from build123d import *

# Parameters (mm, degrees)
BOSS_EXTRUDE1_DEPTH     = 14
SKETCH2_R               = 4
CUT_EXTRUDE1_DEPTH      = 42.386471219
SKETCH3_R               = 6
CUT_EXTRUDE2_DEPTH      = 0.5
CUT_EXTRUDE3_START      = -0.5
SKETCH4_R               = 6
CUT_EXTRUDE3_DEPTH      = 0.5
SKETCH5_R               = 2.5
CUT_EXTRUDE4_DEPTH      = 37.813584449
CUT_EXTRUDE5_REACH      = 43.386
CUT_EXTRUDE5_END_RADIUS = 4
SKETCH7_W               = 0.5
SKETCH7_H               = 14
FILLET1_R               = 2
FILLET2_R               = 0.5
FILLET3_R               = 0.25


with BuildPart() as part:
    # Sketch1 → Boss-Extrude1 (new body)
    with BuildSketch(Plane.XY):
        Polygon((21, 0), (-21, 0), (-21, 6), (-9, 6), (-9, 32.8), (9, 32.8), (9, 6), (21, 6), align=None)
    extrude(amount=BOSS_EXTRUDE1_DEPTH)

    # Sketch2 → Cut-Extrude1 (cut, through all)
    with BuildSketch(Plane.XY.offset(14)):
        with Locations((0, 20)):
            Circle(SKETCH2_R)
    extrude(amount=-CUT_EXTRUDE1_DEPTH, mode=Mode.SUBTRACT)

    # Sketch3 → Cut-Extrude2 (cut)
    with BuildSketch(Plane.XY.offset(14)):
        with Locations((0, 20)):
            Circle(SKETCH3_R)
    extrude(amount=-CUT_EXTRUDE2_DEPTH, mode=Mode.SUBTRACT)

    # Sketch4 → Cut-Extrude3 (cut)
    with BuildSketch(Plane(origin=(0, 0, 0), x_dir=(-1, 0, 0), z_dir=(0, 0, -1)).offset(CUT_EXTRUDE3_START)):
        with Locations(Location((0, 20, 0), (0, 0, 180))):
            Circle(SKETCH4_R)
    extrude(amount=CUT_EXTRUDE3_DEPTH, mode=Mode.SUBTRACT)

    # Sketch5 → Cut-Extrude4 (cut, through all)
    with BuildSketch(Plane(origin=(0, 6, 0), x_dir=(1, 0, 0), z_dir=(0, 1, 0))):
        with Locations(Location((-16, -7, 0), (0, 0, 270))):
            Circle(SKETCH5_R)
        with Locations(Location((16, -7, 0), (0, 0, 90))):
            Circle(SKETCH5_R)
    extrude(amount=-CUT_EXTRUDE4_DEPTH, mode=Mode.SUBTRACT)

    # Cut-Extrude5: up to this cylinder (the profile starts outside it)
    cut_extrude5_end = Plane(origin=(0, 20, 7), z_dir=(0, 0, 1)) * Cylinder(CUT_EXTRUDE5_END_RADIUS, 95.772, mode=Mode.PRIVATE)
    # Sketch7 → Cut-Extrude5 (cut, up to the surface)
    with BuildSketch(Plane(origin=(0, 32.8, 0), x_dir=(1, 0, 0), z_dir=(0, 1, 0)), mode=Mode.PRIVATE) as cut_extrude5_sk1:
        with Locations((0, -7)):
            Rectangle(SKETCH7_W, SKETCH7_H)
    cut_extrude5_tool1 = extrude(cut_extrude5_sk1.sketch, amount=-CUT_EXTRUDE5_REACH, mode=Mode.PRIVATE) - cut_extrude5_end
    add(cut_extrude5_tool1.solids().sort_by_distance((0, 32.8, 7))[0], mode=Mode.SUBTRACT)

    # Fillet1
    fillet1_edges = [part.edges().sort_by_distance(p)[0] for p in [
        (-9, 6, 7),
        (9, 6, 7),
    ]]
    fillet(fillet1_edges, radius=FILLET1_R)

    # Fillet2
    fillet2_edges = [part.edges().sort_by_distance(p)[0] for p in [
        (-9, 32.8, 7),
        (9, 32.8, 7),
        (21, 6, 7),
        (-21, 6, 7),
        (-0.25, 32.8, 7),
        (0.25, 32.8, 7),
    ]]
    fillet(fillet2_edges, radius=FILLET2_R)

    # Fillet3
    fillet3_edges = [part.edges().sort_by_distance(p)[0] for p in [
        (-16, 6, 4.5),
        (16, 6, 9.5),
    ]]
    fillet(fillet3_edges, radius=FILLET3_R)


solid = part.part
Geometry: final body of the model. Coordinates: model frame, mm. A direction names the side the tool comes from. Round coordinates to 2 decimals unless told otherwise and drop trailing zeros. Loops run counter-clockwise (first coordinate to the right, second up) from the corner with the lowest first, then second, coordinate; pieces in that order, holes last.
Q1. Pin query (flat end, axial travel): P1, Ø13, axis at x = 0, y = 20, coming from the -Z side; P2, Ø3, axis at x = -17, z = 10, coming from the +Y side; P3, Ø6.5, axis at y = 29.5, z = 6.5, coming from the +X side; P4, Ø11, axis at x = 0, y = 20, coming from the +Z side. Return the tip coordinate at first contact, or that it passes through.
Q2. Section D-D on z = 1.25. Return loops of the section in (x, y).
Q3. Material intervals for L1, parallel to X at y = 1.9, z = 7; L2, parallel to X at y = 20, z = 0.4; L3, parallel to X at y = 20, z = 5.25, sorted ascending.
Q4. Pull-direction query (Z, two-part tool) for faces 4 (the cylindrical face through (-16.96, 2.92, 9.31)), 5 (the flat face through (5, 32.8, 7)), 6 (the flat face through (0, 9, 14)); classes: released by +Z, released by -Z, zero draft, split by the parting line, or undercut.
Q5. Access query for faces 1 (the flat face through (-16, 6, 4)), 2 (the flat face through (9, 20, 7)), 3 (the flat face through (-1.42, 16.08, 13.5)). Directions: +Z, -Z, +X, -X, +Y, -Y. A direction counts if a zero-diameter tool reaches every point of the face in a straight line with its end or side. Return the directions, or none.
Q6. Section B-B on z = 7. State how many separate pieces and enclosed holes the cut face has, plus the area to 3 significant figures.
Q7. Section A-A on y = 29. Return loops of the section in (x, z), plus the area to 3 significant figures.
Q8. Section C-C on x = -16. Return loops of the section in (y, z).
Evaluation:
1. P1: stops at z = 0
1. P2: stops at y = 6
1. P3: stops at x = 9
1. P4: stops at z = 13.5
2. outline: (-21, 0) - (21, 0) - (21, 5.5) arc R0.5 ccw to (20.5, 6) - (11, 6) arc R2 cw to (9, 8) - (9, 32.3) arc R0.5 ccw to (8.5, 32.8) - (0.75, 32.8) arc R0.5 ccw to (0.25, 32.3) - (0.25, 23.99) arc R4 cw (long way) to (-0.25, 23.99) - (-0.25, 32.3) arc R0.5 ccw to (-0.75, 32.8) - (-8.5, 32.8) arc R0.5 ccw to (-9, 32.3) - (-9, 8) arc R2 cw to (-11, 6) - (-20.5, 6) arc R0.5 ccw to (-21, 5.5) - close
3. L1: x = -21 to -18.5, -13.5 to 13.5, 18.5 to 21
3. L2: x = -9 to -6, 6 to 9
3. L3: x = -9 to -4, 4 to 9
4. face 4: undercut
4. face 5: zero draft
4. face 6: released by +Z
5. face 1: +Z, -Z, -X, +Y
5. face 2: +Z, -Z, +X, +Y
5. face 3: +Z
6. separate pieces: 3
6. enclosed holes: 0
6. area: 621 mm2
7. outline: (-9, 0) - (-0.25, 0) - (-0.25, 14) - (-9, 14) - close; (0.25, 0) - (9, 0) - (9, 14) - (0.25, 14) - close
7. area: 245 mm2
8. outline: (0, 0) - (6, 0) - (6, 4.25) arc R0.25 ccw to (5.75, 4.5) - (0, 4.5) - close; (0, 9.5) - (5.75, 9.5) arc R0.25 ccw to (6, 9.75) - (6, 14) - (0, 14) - close
